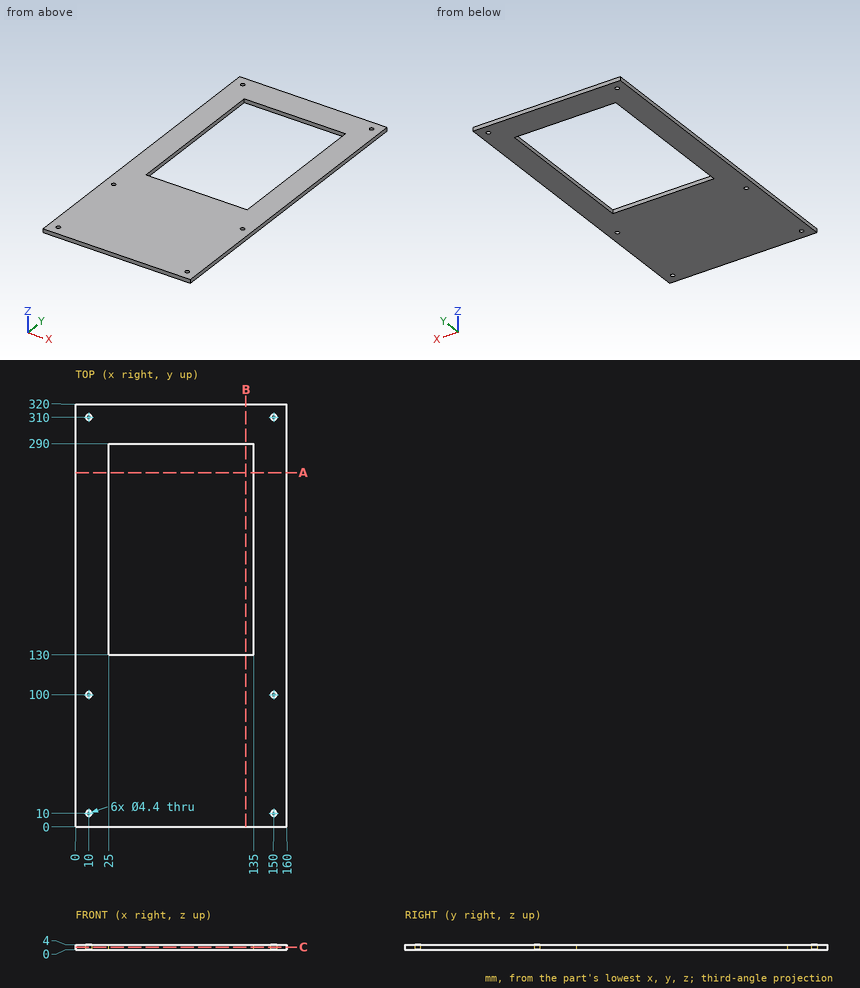
For this review, use the dimensioned drawing (mm, ordinates from the lowest corner) and the shaded views. Coordinates: 2 decimals unless noted, no trailing zeros. Loops run counter-clockwise (first coordinate to the right, second up) from the corner with the lowest first, then second, coordinate; pieces in that order, holes last. Notation, with made-up numbers: (25.25, 71.5) -> (77.25, 71.5) arc R14 cw to (77.25, 86.5) -> close; hole circle Ø11 at (83, -6.75). An arc over 180 degrees is marked (long way). Use a Markdown table: item, result. Add a question column.
Item 1: We need section B-B, the plane x = 129. Write out the cut boundary in (y, z).
Item 2: Wall thickness on L1, parallel to Y at x = 150, z = 1.5; L2, parallel to Y at x = 32, z = 1.1; L3, parallel to X at y = 310, z = 2.25: over which ranges is each line inside the solid? List them lowest first. Write a range as from..to.
Item 3: We need section A-A, the plane y = 268. Write out the cut boundary in (x, z).
Item 4: Clearance check with a flat-ended pin moving along its axis: P1, Ø7, axis at x = 150, y = 10, coming from the -Z side. State where the tip first meets the part, or that it passes through.
Item 5: We need section C-C, the plane z = 2.2. Write out the cut boundary in (x, y), and give its area (3 significant figures).
Numbers:
| question | item | result |
|---|---|---|
| 1 | outline | (0, 0) -> (130, 0) -> (130, 4) -> (0, 4) -> close; (290, 0) -> (320, 0) -> (320, 4) -> (290, 4) -> close |
| 2 | L1 | y = 0..7.8, 12.2..97.8, 102.2..307.8, 312.2..320 |
| 2 | L2 | y = 0..130, 290..320 |
| 2 | L3 | x = 0..7.8, 12.2..147.8, 152.2..160 |
| 3 | outline | (0, 0) -> (25, 0) -> (25, 4) -> (0, 4) -> close; (135, 0) -> (160, 0) -> (160, 4) -> (135, 4) -> close |
| 4 | P1 | stops at z = 0 |
| 5 | outline | (0, 0) -> (160, 0) -> (160, 320) -> (0, 320) -> close; hole circle Ø4.4 at (10, 10); hole circle Ø4.4 at (10, 100); hole circle Ø4.4 at (10, 310); hole (25, 130) -> (135, 130) -> (135, 290) -> (25, 290) -> close; hole circle Ø4.4 at (150, 10); hole circle Ø4.4 at (150, 100); hole circle Ø4.4 at (150, 310) |
| 5 | area | 33,500 mm^2 |
